Here's the drawing with two shaded views (mm, measured from the low corner). I have some questions. A direction names the side the tool comes from. Give positions to 0.01 mm unless a question says otherwise; leave off trailing zeros. Write each loop counter-clockwise with the first axis right and the second up, starting at its lowest first coordinate (ties: lowest second). Pieces come first, ordered by that corner, then holes. Notation, with made-up numbers: (-1.5, -1.5) - (44.5, -1.5) arc R17 cw to (44.5, 21.5) - close; hole circle Ø4 at (57, 10). An arc over 180 degrees is marked (long way). Write item = value, one per line.
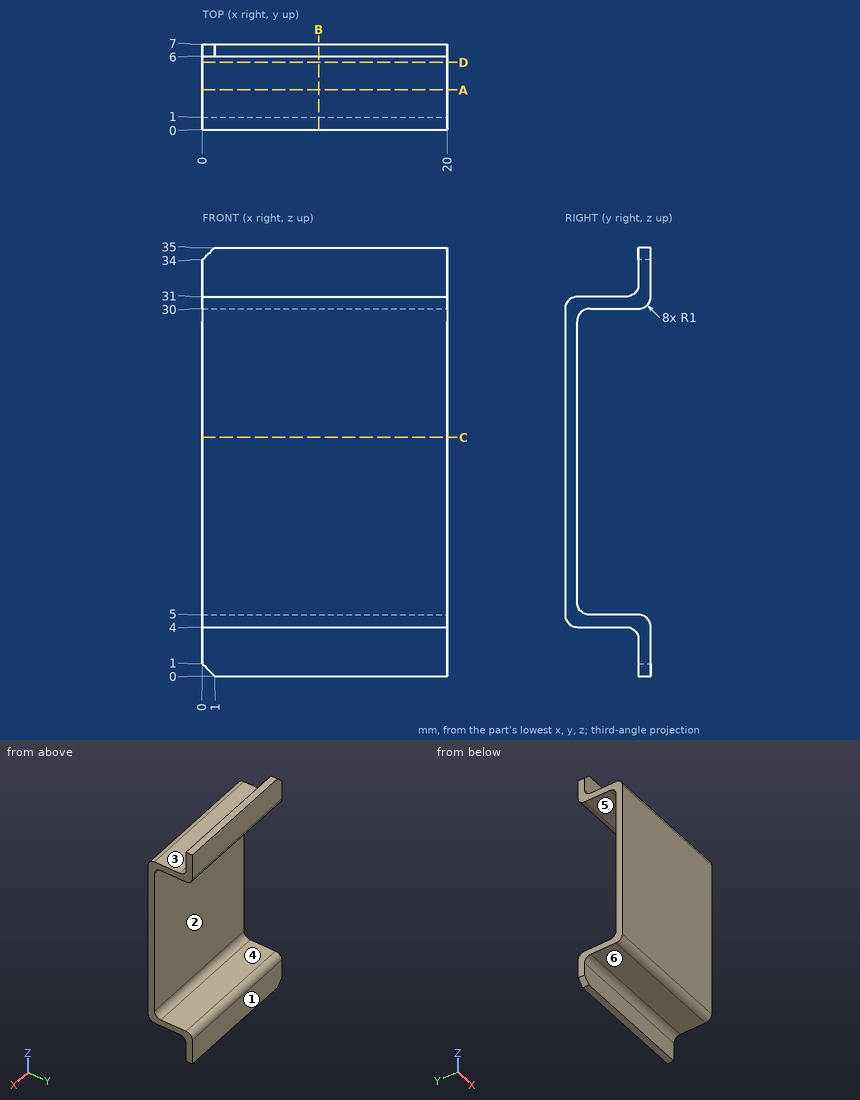
1. I need wall thicknesses on line 1 (Z direction, x = 9.75, y = 5); line 2 (Y direction, x = 7.5, z = 33.5); line 3 (Y direction, x = 1.5, z = 21). Which ranges of each line are inside material? Lowest first, please.
Filled sheet:
line_1 = 4 to 5, 30 to 31
line_2 = 6 to 7
line_3 = 0 to 1
2. If we section it at C-C, the plane z = 19.5: Please give me the cut outline in (x, y).
Filled sheet:
outline = (0, 0) - (20, 0) - (20, 1) - (0, 1) - close
3. If we section it at A-A, the plane y = 3.25: Please give me the cut outline in (x, z).
Filled sheet:
outline = (0, 4) - (20, 4) - (20, 5) - (0, 5) - close; (0, 30) - (20, 30) - (20, 31) - (0, 31) - close
4. Thinking about a two-plate mould opening in Z: for the marked faces 3, 4, 5 and 6, which applies, pulls with the +Z half, pulls with the -Z half, needs draft (parallel to the pull), parting line crosses it, or undercut?
Filled sheet:
face_3 = pulls with the +Z half
face_4 = undercut
face_5 = undercut
face_6 = pulls with the -Z half
5. If we section it at B-B, the plane x = 9.5: Please give me the cut outline in (y, z), and give its area (3 significant figures).
Filled sheet:
outline = (0, 5) arc R1 ccw to (1, 4) - (5, 4) arc R1 cw to (6, 3) - (6, 0) - (7, 0) - (7, 4) arc R1 ccw to (6, 5) - (2, 5) arc R1 cw to (1, 6) - (1, 29) arc R1 cw to (2, 30) - (6, 30) arc R1 ccw to (7, 31) - (7, 35) - (6, 35) - (6, 32) arc R1 cw to (5, 31) - (1, 31) arc R1 ccw to (0, 30) - close
area = 47.0 mm2
6. If we section it at D-D, the plane y = 5.5: Please give me the cut outline in (x, z), and give its area (3 significant figures).
Filled sheet:
outline = (0, 3.87) - (20, 3.87) - (20, 5) - (0, 5) - close; (0, 30) - (20, 30) - (20, 31.13) - (0, 31.13) - close
area = 45.4 mm2
7. Which directions (+Z, -Z, +X, -X, +Y, -Y) give clear straight access to the entire face, cutting with the end or side of a thin tool? Please do the marked faces 1 and 2.
Filled sheet:
face_1 = +Z, -Z, +X, -X, +Y
face_2 = +X, -X, +Y
8. For pin 1 (1.2 mm diameter, centred on x = 7.5, y = 3.5, fed in from +Z); pin 2 (3 mm diameter, centred on x = 8, y = 2, fed in from -Z); pin 3 (1.2 mm diameter, centred on x = 6.5, y = 5, fed in from -Z), each with a flat end and sliding along its axis, tell me the tip position at first contact or that it passes through.
Filled sheet:
pin_1 = 31
pin_2 = 4
pin_3 = 3.8
